Check sheet for the modelled part. Datum: model origin and axes. Units: mm. Face numbers are marked on the shaded views. Give positions to 0.01 mm unless a question says otherwise; leave off trailing zeros. Order: outer loops, then holes, each group sorted by start corner. A loop starts at its lowest first (then second) coordinate and runs counter-clockwise, first axis right, second up. Notation, with made-up numbers: (11, 12.25) -> (48, 12.25) arc R17 ccw to (48, 34.25) -> close; hole circle Ø1 at (16.5, -7.75). An arc over 180 degrees is marked (long way). Answer in a Markdown table with one row per item. Add a question column.
(1) Go/stop test with a flat-tipped pin: pin 1 (8 mm diameter, centred on y = -5, z = 9.5, fed in from -X). Record where the tip stops, or that it passes through.
(2) Cross-section at B-B (z = 10). State how many separate pieces and enclosed holes the cut face has, then the cut area to 3 significant figures.
(3) Release check for a two-part mould opening along Z. For the marked faces 1, 2, 3 and 4 record: released by +Z, released by -Z, zero draft, split by the parting line, or undercut.
(4) Cross-section at A-A (x = 0). Record the cut outline in (y, z) (1 decimal), then the cut area to 3 significant figures.
(5) Thickness scan on L1, parallel to Y at x = 0, z = 7.75; L2, parallel to Z at x = -5.75, y = -1.5; L3, parallel to Y at x = 0, z = 12.5. Record the ranges inside material, lowest first. Write a range as [from, to].
```python
from build123d import *

# Parameters (mm, degrees)
SKETCH1_R           = 4.7625
BOSS_EXTRUDE1_DEPTH = 16.256
SKETCH2_R           = 4.7625
CUT_EXTRUDE1_DEPTH  = 16.256
CHAMFER1_SIZE       = 0.396875


with BuildPart() as part:
    # Sketch1 → Boss-Extrude1 (new body)
    with BuildSketch(Plane.XY):
        with BuildLine():
            Line((-8.128, 9.525), (-8.128, -9.525))
            Line((-8.128, -9.525), (8.128, -9.525))
            Line((8.128, -9.525), (8.128, 9.525))
            ThreePointArc((8.128, 9.525), (0, 17.653), (-8.128, 9.525))
        make_face()
        with Locations((0, 9.525)):
            Circle(SKETCH1_R, mode=Mode.SUBTRACT)
    extrude(amount=BOSS_EXTRUDE1_DEPTH)

    # Sketch2 → Cut-Extrude1 (cut)
    with BuildSketch(Plane(origin=(8.128, 0, 0), x_dir=(0, 0, -1), z_dir=(1, 0, 0))):
        with BuildLine():
            ThreePointArc((0, -1.397), (-2.380636089, -7.144363924), (-8.128000019, -9.525))
            Line((-8.128000019, -9.525), (0, -9.525))
            Line((0, -9.525), (0, -1.397))
        make_face()
        with BuildLine():
            ThreePointArc((-8.128000019, -9.525), (-13.875363924, -7.144363911), (-16.256, -1.397))
            Line((-16.256, -1.397), (-16.256, -9.525))
            Line((-16.256, -9.525), (-8.128000019, -9.525))
        make_face()
        with Locations(Location((-8.128, -1.397, 0), (0, 0, 90))):
            Circle(SKETCH2_R)
    extrude(amount=-CUT_EXTRUDE1_DEPTH, mode=Mode.SUBTRACT)

    # Chamfer1
    chamfer1_edges = [part.edges().sort_by_distance(p)[0] for p in [
        (-4.7625, 9.525, 16.256),
        (-8.128, 4.064, 16.256),
        (8.128, 4.064, 16.256),
        (8.128, -9.525, 8.128),
        (-8.128, -9.525, 8.128),
        (8.128, 4.064, 0),
        (8.128, -6.1595, 8.128),
        (-8.128, -6.1595, 8.128),
        (-8.128, 4.064, 0),
        (0, 17.653, 0),
        (0, 17.653, 16.256),
    ]]
    chamfer(chamfer1_edges, length=CHAMFER1_SIZE)


solid = part.part
```
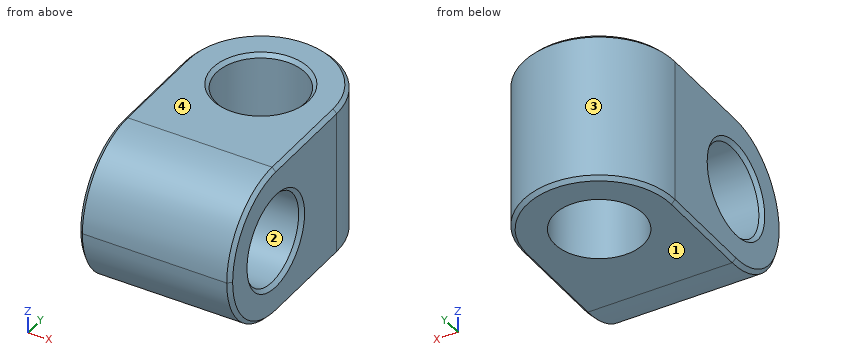
Answer below:
| question | item | result |
|---|---|---|
| 1 | pin 1 | stops at x = -8.13 |
| 2 | separate pieces | 2 |
| 2 | enclosed holes | 1 |
| 2 | area | 196 mm² |
| 3 | face 1 | released by -Z |
| 3 | face 2 | undercut |
| 3 | face 3 | zero draft |
| 3 | face 4 | released by +Z |
| 4 | outline | (-1.4, 0) -> (4.8, 0) -> (4.8, 15.9) -> (4.4, 16.3) -> (-1.4, 16.3) arc R8.1 ccw to start; (14.3, 0) -> (17.3, 0) -> (17.7, 0.4) -> (17.7, 15.9) -> (17.3, 16.3) -> (14.7, 16.3) -> (14.3, 15.9) -> close; hole circle Ø9.5 at (-1.4, 8.1) |
| 4 | area | 187 mm² |
| 5 | L1 | y = [-9.52, -6.14], [3.35, 4.76], [14.29, 17.65] |
| 5 | L2 | z = [0, 3.37], [12.89, 16.26] |
| 5 | L3 | y = [-8.25, -3.29], [0.49, 4.76], [14.29, 17.65] |
